from build123d import *

# Parameters (mm, degrees)
F0_W     = 79
F0_H     = 59
F0_W_2   = 75
F0_H_2   = 55
F1_DEPTH = 4
F2_DEPTH = 31
F3_DEPTH = 33
F4_R     = 8.5
F5_DEPTH = 41.501


# Not quite as in the source:
# - a feature names something its author has since deleted; it is built from what else it names


with BuildPart() as f1:
    # F0 (on Top) → F1 (new body)
    with BuildSketch(Plane.XY):
        Polygon((41.5, -31.5), (41.5, 31.5), (7.5, 31.5), (3.5, 31.5), (-3.5, 31.5), (-7.5, 31.5), (-41.5, 31.5), (-41.5, -31.5), (-7.5, -31.5), (-3.5, -31.5), (3.5, -31.5), (7.5, -31.5), align=None)
        Rectangle(F0_W, F0_H, mode=Mode.SUBTRACT)
        Rectangle(F0_W, F0_H)
        Rectangle(F0_W_2, F0_H_2, mode=Mode.SUBTRACT)
        Rectangle(F0_W_2, F0_H_2)
        with BuildLine():
            ThreePointArc((-7.5, -31.5), (0, -39), (7.5, -31.5))
            Line((7.5, -31.5), (3.5, -31.5))
            ThreePointArc((3.5, -31.5), (0, -35), (-3.5, -31.5))
            Line((-3.5, -31.5), (-7.5, -31.5))
        make_face()
        with BuildLine():
            Line((3.5, 31.5), (7.5, 31.5))
            ThreePointArc((7.5, 31.5), (0, 39), (-7.5, 31.5))
            Line((-7.5, 31.5), (-3.5, 31.5))
            ThreePointArc((-3.5, 31.5), (0, 35), (3.5, 31.5))
        make_face()
    extrude(amount=F1_DEPTH)

    # F0 (on Top) → F2 (join)
    with BuildSketch(Plane.XY):
        Rectangle(F0_W, F0_H)
        Rectangle(F0_W_2, F0_H_2, mode=Mode.SUBTRACT)
    extrude(amount=F2_DEPTH)

    # F0 (on Top) → F3 (join)
    with BuildSketch(Plane.XY):
        Polygon((41.5, -31.5), (41.5, 31.5), (7.5, 31.5), (3.5, 31.5), (-3.5, 31.5), (-7.5, 31.5), (-41.5, 31.5), (-41.5, -31.5), (-7.5, -31.5), (-3.5, -31.5), (3.5, -31.5), (7.5, -31.5), align=None)
        Rectangle(F0_W, F0_H, mode=Mode.SUBTRACT)
    extrude(amount=F3_DEPTH)

    # F4 (on Right) → F5 (cut, through all)
    with BuildSketch(Plane.YZ):
        with Locations((0, 14)):
            Circle(F4_R)
    extrude(amount=-F5_DEPTH, mode=Mode.SUBTRACT)


solid = f1.part
Could you check a few things on this model? Use its own coordinates, in mm. A direction names the side the tool comes from. Round coordinates to 2 decimals unless told otherwise and drop trailing zeros. Order: outer loops, then holes, each group sorted by start corner. A loop starts at its lowest first (then second) coordinate and runs counter-clockwise, first axis right, second up.
Q1. I'm going to push flat-ended pins straight in: P1, Ø1.6, axis at x = 18, z = 32, coming from the +Y side; P2, Ø8, axis at x = -4, y = 16.5, coming from the +Z side; P3, Ø8, axis at x = -28.5, y = 26, coming from the -Z side; P4, Ø8, axis at x = 1.5, z = 20, coming from the -Y side. Where does each tip first touch, or does it pass through?
Geometry says:
P1: stops at y = 31.5
P2: stops at z = 4
P3: stops at z = 0
P4: stops at y = -31.5
Q2. Imagine slicing it at D-D, the plane y = 0. List the corners of the cut face in (x, z) for me, then the cut area to 3 significant figures.
Geometry says:
outline: (-41.5, 0) - (41.5, 0) - (41.5, 33) - (39.5, 33) - (39.5, 31) - (37.5, 31) - (37.5, 4) - (-37.5, 4) - (-37.5, 5.5) - (-41.5, 5.5) - close; (-41.5, 22.5) - (-37.5, 22.5) - (-37.5, 31) - (-39.5, 31) - (-39.5, 33) - (-41.5, 33) - close
area: 488 mm2
Q3. Imagine slicing it at C-C, the plane y = 15. List the corners of the cut face in (x, z) for me.
Geometry says:
outline: (-41.5, 0) - (41.5, 0) - (41.5, 33) - (39.5, 33) - (39.5, 31) - (37.5, 31) - (37.5, 4) - (-37.5, 4) - (-37.5, 31) - (-39.5, 31) - (-39.5, 33) - (-41.5, 33) - close
Q4. Please list where these lines run through material, in increasing order: probe 1 along Y at (x, z) = (19, 28); probe 2 along X at (y, z) = (-19, 16.5); probe 3 along Z at (x, y) = (-40.05, 0).
Geometry says:
probe 1: y = -31.5 to -27.5, 27.5 to 31.5
probe 2: x = -41.5 to -37.5, 37.5 to 41.5
probe 3: z = 0 to 5.5, 22.5 to 33
Q5. Imagine slicing it at B-B, the plane z = 3. List the corners of the cut face in (x, y) for me.
Geometry says:
outline: (-41.5, -31.5) - (-7.5, -31.5) arc R7.5 ccw to (7.5, -31.5) - (41.5, -31.5) - (41.5, 31.5) - (7.5, 31.5) arc R7.5 ccw to (-7.5, 31.5) - (-41.5, 31.5) - close; hole (-3.5, -31.5) arc R3.5 ccw to (3.5, -31.5) - close; hole (-3.5, 31.5) - (3.5, 31.5) arc R3.5 ccw to start
Q6. Which directions (+Z, -Z, +X, -X, +Y, -Y) give clear straight access to the entire face, cutting with the end or side of a thin tool? Please do faces 5 (the face through (-1, 29.5, 32)), 6 (the face through (-1, 1, 0)), 7 (the face through (-39.47, -1.84, 5.7)), 8 (the face through (-0.1, 35.3, 4)), 9 (the face through (0, -35, 2)).
Geometry says:
face 5: +Z
face 6: -Z, +X, -X, +Y, -Y
face 7: -X
face 8: +Z, +X, -X, +Y
face 9: +Z, -Z
Q7. Thinking about a two-plate mould opening in Y: for faces 1 (the face through (39.5, 0, 32)), 2 (the face through (-37.5, 0, 23)), 3 (the face through (0, 39, 2)), 4 (the face through (-3, -30, 33)), which applies, released by +Y, released by -Y, zero draft, split by the parting line, or undercut?
Geometry says:
face 1: undercut
face 2: undercut
face 3: released by +Y
face 4: zero draft
Q8. Imagine slicing it at A-A, the plane x = 0. List the corners of the cut face in (y, z) for me, then the cut area to 3 significant figures.
Geometry says:
outline: (-39, 0) - (-35, 0) - (-35, 4) - (-39, 4) - close; (-31.5, 0) - (31.5, 0) - (31.5, 33) - (29.5, 33) - (29.5, 31) - (27.5, 31) - (27.5, 4) - (-27.5, 4) - (-27.5, 31) - (-29.5, 31) - (-29.5, 33) - (-31.5, 33) - close; (35, 0) - (39, 0) - (39, 4) - (35, 4) - close
area: 508 mm2
